CAD build for the part. Positions are in the model's coordinates, mm. Round coordinates to 2 decimals unless told otherwise and drop trailing zeros. Order: outer loops, then holes, each group sorted by start corner. A loop starts at its lowest first (then second) coordinate and runs counter-clockwise, first axis right, second up. Notation, with made-up numbers: M 28,15.25 L 36,15.25 A22 cw 36,53.25 Z; hole C 1.25,-1 d4. An arc over 180 degrees is marked long. Answer as a JSON object with one key per item and string values. Group by question number.
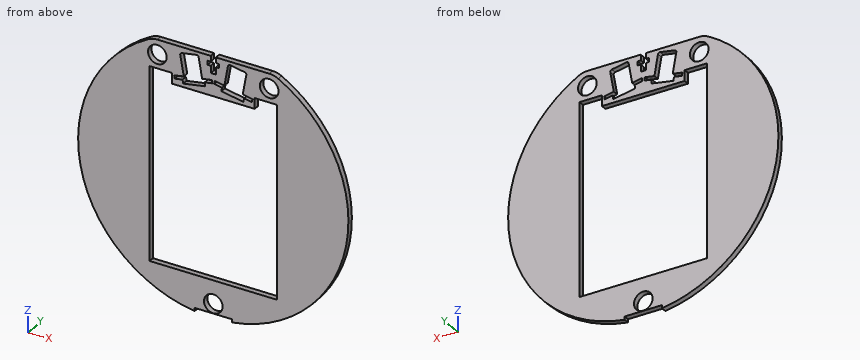
```python
from build123d import *

# Parameters (mm, degrees)
BOSS_EXTRUDE1_DEPTH = 3
CUT_EXTRUDE1_DEPTH  = 103.574363269
CUT_EXTRUDE3_DEPTH  = 103.574363269
CUT_EXTRUDE4_DEPTH  = 103.574363269
SKETCH6_W           = 68.4
SKETCH6_H           = 3
CUT_EXTRUDE5_DEPTH  = 103.574363269
SKETCH7_R           = 5
CUT_EXTRUDE6_DEPTH  = 103.574363269
SKETCH11_R          = 5
CUT_EXTRUDE10_DEPTH = 103.574363269
SKETCH15_W          = 20
SKETCH15_H          = 1.7
CUT_EXTRUDE14_DEPTH = 103.574363269
CUT_EXTRUDE15_DEPTH = 103.085748271


with BuildPart() as part:
    # Sketch1 → Boss-Extrude1 (new body)
    with BuildSketch(Plane(origin=(0, 0, 0), x_dir=(1, 0, 0), z_dir=(0, 1, 0))):
        with BuildLine():
            Line((-30.029977361, -64.812867647), (30.029977361, -64.812867647))
            ThreePointArc((30.029977361, -64.812867647), (32.509837414, -64.500503794), (34.834773739, -63.582926471))
            ThreePointArc((34.834773739, -63.582926471), (0, 72.5), (-34.834773739, -63.582926471))
            ThreePointArc((-34.834773739, -63.582926471), (-32.509837414, -64.500503794), (-30.029977361, -64.812867647))
        make_face()
    extrude(amount=BOSS_EXTRUDE1_DEPTH)

    # Sketch2 → Cut-Extrude1 (cut, through all)
    with BuildSketch(Plane(origin=(0, 3, 0), x_dir=(1, 0, 0), z_dir=(0, 1, 0))):
        Polygon((-34.2, -49.675685802), (-22.2, -49.675685802), (-22.2, -44), (22.2, -44), (22.2, -49.675685802), (34.2, -49.675685802), (34.2, 49.675685802), (22.2, 49.675685802), (22.2, 44), (-22.2, 44), (-22.2, 49.675685802), (-34.2, 49.675685802), align=None)
    extrude(amount=-CUT_EXTRUDE1_DEPTH, mode=Mode.SUBTRACT)

    # Sketch4 → Cut-Extrude3 (cut, through all)
    with BuildSketch(Plane(origin=(0, 3, 0), x_dir=(1, 0, 0), z_dir=(0, 1, 0))):
        Polygon((-20.983760839, -48.753080005), (-0.795201902, -52.312867647), (-0.5, -50.638694467), (-20.688558937, -47.078906825), align=None)
        Polygon((20.983760839, -48.753080005), (20.688558937, -47.078906825), (0.5, -50.638694467), (0.795201902, -52.312867647), align=None)
    extrude(amount=-CUT_EXTRUDE3_DEPTH, mode=Mode.SUBTRACT)

    # Sketch5 → Cut-Extrude4 (cut, through all)
    with BuildSketch(Plane(origin=(0, 3, 0), x_dir=(1, 0, 0), z_dir=(0, 1, 0))):
        with BuildLine():
            Line((5.965442605, -51.401214714), (15.813520135, -49.664732938))
            Line((15.813520135, -49.664732938), (17.72365009, -60.497618221))
            ThreePointArc((17.72365009, -60.497618221), (17.557994381, -61.244842835), (16.912490514, -61.656074151))
            Line((16.912490514, -61.656074151), (9.03402849, -63.045259573))
            ThreePointArc((9.03402849, -63.045259573), (8.286803876, -62.879603864), (7.87557256, -62.234099997))
            Line((7.87557256, -62.234099997), (5.965442605, -51.401214714))
        make_face()
        Polygon((16.503125986, -47.81691158), (4.68543295, -49.900689712), (4.338136595, -47.931074206), (16.155829631, -45.847296074), align=None)
        Polygon((-16.155829631, -45.847296074), (-4.338136595, -47.931074206), (-4.68543295, -49.900689712), (-16.503125986, -47.81691158), align=None)
        with BuildLine():
            Line((-9.03402849, -63.045259573), (-16.912490514, -61.656074151))
            ThreePointArc((-16.912490514, -61.656074151), (-17.557994381, -61.244842835), (-17.72365009, -60.497618221))
            Line((-17.72365009, -60.497618221), (-15.813520135, -49.664732938))
            Line((-15.813520135, -49.664732938), (-5.965442605, -51.401214714))
            Line((-5.965442605, -51.401214714), (-7.87557256, -62.234099997))
            ThreePointArc((-7.87557256, -62.234099997), (-8.286803876, -62.879603864), (-9.03402849, -63.045259573))
        make_face()
    extrude(amount=-CUT_EXTRUDE4_DEPTH, mode=Mode.SUBTRACT)

    # Sketch6 → Cut-Extrude5 (cut, through all)
    with BuildSketch(Plane(origin=(0, 3, 0), x_dir=(1, 0, 0), z_dir=(0, 1, 0))):
        with Locations((0, 51.175685802)):
            Rectangle(SKETCH6_W, SKETCH6_H)
    extrude(amount=-CUT_EXTRUDE5_DEPTH, mode=Mode.SUBTRACT)


with BuildPart() as cut_extrude5_kept_piece:
    # of the separate pieces the step leaves, the one the design keeps (cut_extrude5_pieces_kept)
    add(part.part.solids().sort_by_distance((-34.834773739, 0, 63.582926471))[0])

    # Sketch7 → Cut-Extrude6 (cut, through all)
    with BuildSketch(Plane(origin=(0, 3, 0), x_dir=(1, 0, 0), z_dir=(0, 1, 0))):
        with Locations(Location((-30, -57, 0), (0, 0, 90))):
            Circle(SKETCH7_R)
        with Locations(Location((30, -57, 0), (0, 0, 270))):
            Circle(SKETCH7_R)
    extrude(amount=-CUT_EXTRUDE6_DEPTH, mode=Mode.SUBTRACT)

    # Sketch11 → Cut-Extrude10 (cut, through all)
    with BuildSketch(Plane(origin=(0, 3, 0), x_dir=(1, 0, 0), z_dir=(0, 1, 0))):
        with Locations(Location((0, 65, 0), (0, 0, 270))):
            Circle(SKETCH11_R)
    extrude(amount=-CUT_EXTRUDE10_DEPTH, mode=Mode.SUBTRACT)

    # Sketch15 → Cut-Extrude14 (cut, through all)
    with BuildSketch(Plane(origin=(0, 3, 0), x_dir=(1, 0, 0), z_dir=(0, 1, 0))):
        with Locations((0, 70.957033082)):
            Rectangle(SKETCH15_W, SKETCH15_H)
    extrude(amount=-CUT_EXTRUDE14_DEPTH, mode=Mode.SUBTRACT)


with BuildPart() as body_2:
    # of the pieces the cut leaves, the one that is kept (cut_extrude14_keep)
    add(cut_extrude5_kept_piece.part.solids().sort_by_distance((-34.834773739, 0, 63.582926471))[0])

    # Sketch16 → Cut-Extrude15 (cut, through all)
    with BuildSketch(Plane(origin=(0, 3, 0), x_dir=(1, 0, 0), z_dir=(0, 1, 0))):
        Polygon((-1.35, -64.812867647), (1.35, -64.812867647), (1.35, -61.812867647), (3.1, -61.812867647), (3.1, -59.612867647), (1.35, -59.612867647), (1.35, -55.812867647), (-1.35, -55.812867647), (-1.35, -59.612867647), (-3.1, -59.612867647), (-3.1, -61.812867647), (-1.35, -61.812867647), align=None)
    extrude(amount=-CUT_EXTRUDE15_DEPTH, mode=Mode.SUBTRACT)


solid = body_2.part
```
Item 1: Cut at A-A, the plane x = -32.5. Give the cut face in (y, z), and give its area (3 significant figures).
Item 2: Cut at D-D, the plane y = 1.4. Give the number of separate pieces and of enclosed holes in the cut face, and give its area (3 significant figures).
Item 3: Cut at B-B, the plane z = -47.5. Give the cut face in (x, y), and give its area (3 significant figures).
Item 4: Drill centre lines: line 1 (Z direction, x = -20, y = 2.65); line 2 (X direction, y = 1.45, z = 57); line 3 (Z direction, x = -34, y = 1.8). Where is each one in solid material? Low to high. Write a range as [from, to].
Item 5: Flat gauge pins, fed straight in: pin 1 Ø0.9 at (x, y) = (-26.5, 2) entering from -Z; pin 2 Ø0.9 at (x, y) = (4, 1) entering from -Z; pin 3 Ø0.8 at (x, y) = (-0.5, 1.5) entering from +Z. Where does each tip first touch, or does it go through?
Item 6: Cut at C-C, the plane z = 19. Give the cut face in (x, y).
Response values:
{
 "1": {"outline": "M 0,-64.81 L 3,-64.81 L 3,-52.68 L 0,-52.68 Z; M 0,49.68 L 3,49.68 L 3,52.67 L 0,52.67 Z; M 0,61.33 L 3,61.33 L 3,64.5 L 0,64.5 Z", "area": "54.9 mm^2"},
 "2": {"separate pieces": "1", "enclosed holes": "6", "area": "8,760 mm^2"},
 "3": {"outline": "M -54.77,0 L -34.2,0 L -34.2,3 L -54.77,3 Z; M 34.2,0 L 54.77,0 L 54.77,3 L 34.2,3 Z", "area": "123 mm^2"},
 "4": {"line 1": "[-69.69, -52.68], [44, 47.2], [48.93, 64.81]", "line 2": "[-44.8, -35], [-25, -17.11], [-6.95, -1.35], [1.35, 6.95], [17.11, 25], [35, 44.8]", "line 3": "[-64.03, -52.68], [49.68, 54], [60, 63.99]"},
 "5": {"pin 1": "z = -67.66", "pin 2": "z = -70.11", "pin 3": "z = 55.81"},
 "6": {"outline": "M -69.97,0 L -34.2,0 L -34.2,3 L -69.97,3 Z; M 34.2,0 L 69.97,0 L 69.97,3 L 34.2,3 Z"}
}
